from build123d import *

# Parameters (mm, degrees)
SKETCH1_R           = 1.05
BOSS_EXTRUDE1_DEPTH = 1.5
FILLET1_R           = 1.5


with BuildPart() as part:
    # Sketch1 → Boss-Extrude1 (new body)
    with BuildSketch(Plane(origin=(0, 0, 0), x_dir=(0, 0, -1), z_dir=(1, 0, 0))):
        Polygon((0, 0), (0, 75.5), (21.5, 75.5), (40, 0), (35.881667859, 0), (29.755840045, 25), (4, 25), (4, 0), align=None)
        with Locations((5.5, 72.5)):
            Circle(SKETCH1_R, mode=Mode.SUBTRACT)
        with Locations((18.5, 72.5)):
            Circle(SKETCH1_R, mode=Mode.SUBTRACT)
        Polygon((4, 69.5), (18.851866535, 69.5), (4, 29), align=None, mode=Mode.SUBTRACT)
        Polygon((8.260475549, 29), (20.558388216, 62.535546651), (28.775707595, 29), align=None, mode=Mode.SUBTRACT)
    extrude(amount=BOSS_EXTRUDE1_DEPTH)

    # Fillet1
    fillet1_edges = [part.edges().sort_by_distance(p)[0] for p in [
        (0.75, 75.5, -21.5),
        (0.75, 25, -29.755840045),
        (0.75, 25, -4),
        (0.75, 69.5, -4),
        (0.75, 29, -4),
        (0.75, 69.5, -18.851866535),
        (0.75, 29, -8.260475549),
        (0.75, 29, -28.775707595),
        (0.75, 62.535546651, -20.558388216),
    ]]
    fillet(fillet1_edges, radius=FILLET1_R)


solid = part.part
Input: part model. Units: mm. Frame: model coordinates. A direction names the side the tool comes from. Coordinates: 2 decimals unless noted, no trailing zeros. Loops run counter-clockwise (first coordinate to the right, second up) from the corner with the lowest first, then second, coordinate; pieces in that order, holes last. Notation, with made-up numbers: (36, 37) - (66, 37) arc R8 cw to (66, 48) - close; hole circle Ø8 at (29, 72). An arc over 180 degrees is marked (long way). Answer in a Markdown table with one row per item. Add a question column.
Item 1: Section query C-C on z = -8. Return the cut outline in (x, y), then the cut area to 3 significant figures.
Item 2: Line query: line 1 along Y through (x, z) = (0.6, -5.5); line 2 along Z through (x, y) = (0.95, 43); line 3 along Z through (x, y) = (0.9, 48.5). Output: solid intervals per line, ascending. Write a range as [from, to].
Item 3: Section query D-D on y = 7.5. Return the cut outline in (x, z), then the cut area to 3 significant figures.
Item 4: Contact query for a flat-ended pin moving along its axis: P1, Ø0.8, axis at x = 1, y = 52.5, coming from the -Z side. Output: stop coordinate, or through.
Item 5: Mould query, pull axis Y, two halves, no side actions, for faces 1 (the cylindrical face through (0.76, 29.589, -28.056)), 2 (the flat face through (1, 0, -38)), 3 (the flat face through (1, 37, 0)), 4 (the cylindrical face through (0.76, 75.189, -21.238)). Classes: released by +Y, released by -Y, zero draft, split by the parting line, or undercut.
Item 6: Access query for faces 5 (the cylindrical face through (0.76, 35.976, -5.209)), 6 (the flat face through (0, 44, -11)), 7 (the cylindrical face through (0.76, 24.69, -29.49)). Directions: +Z, -Z, +X, -X, +Y, -Y. A direction counts if a zero-diameter tool reaches every point of the face in a straight line with its end or side. Return the directions, or none.
Item 7: Section query B-B on y = 45. Return the cut outline in (x, z).
Item 8: Section query A-A on x = 0.9. Return the cut outline in (y, z), then the cut area to 3 significant figures.
Recorded:
| question | item | result |
|---|---|---|
| 1 | outline | (0, 25) - (1.5, 25) - (1.5, 39.91) - (0, 39.91) - close; (0, 69.5) - (1.5, 69.5) - (1.5, 75.5) - (0, 75.5) - close |
| 1 | area | 31.4 mm^2 |
| 2 | line 1 | [25, 35.95], [69.5, 71.45], [73.55, 75.5] |
| 2 | line 2 | [-29.46, -25.35], [-13.39, -9.13], [-4, 0] |
| 2 | line 3 | [-28.12, -24], [-15.41, -11.15], [-4, 0] |
| 3 | outline | (0, -38.16) - (1.5, -38.16) - (1.5, -34.04) - (0, -34.04) - close; (0, -4) - (1.5, -4) - (1.5, 0) - (0, 0) - close |
| 3 | area | 12.2 mm^2 |
| 4 | P1 | z = -27.23 |
| 5 | face 1 | undercut |
| 5 | face 2 | released by -Y |
| 5 | face 3 | zero draft |
| 5 | face 4 | released by +Y |
| 6 | face 5 | +X, -X |
| 6 | face 6 | +Z, -Z, -X, +Y, -Y |
| 6 | face 7 | +X, -X, -Y |
| 7 | outline | (0, -28.97) - (1.5, -28.97) - (1.5, -24.86) - (0, -24.86) - close; (0, -14.13) - (1.5, -14.13) - (1.5, -9.87) - (0, -9.87) - close; (0, -4) - (1.5, -4) - (1.5, 0) - (0, 0) - close |
| 8 | outline | (0, -40) - (74.36, -21.78) arc R1.5 ccw to (75.5, -20.32) - (75.5, 0) - (0, 0) - (0, -4) - (23.5, -4) arc R1.5 cw to (25, -5.5) - (25, -28.58) arc R1.5 cw to (23.86, -30.04) - (0, -35.88) - close; hole (29, -26.86) arc R1.5 ccw to (30.86, -28.32) - (57.76, -21.73) arc R1.5 ccw to (57.92, -18.86) - (31.02, -9) arc R1.5 ccw to (29, -10.41) - close; hole (36.93, -6.91) - (67.48, -18.11) arc R1.5 ccw to (69.5, -16.7) - (69.5, -5.5) arc R1.5 ccw to (68, -4) - (37.45, -4) arc R1.5 ccw to start; hole circle Ø2.1 at (72.5, -18.5); hole circle Ø2.1 at (72.5, -5.5) |
| 8 | area | 967 mm^2 |
